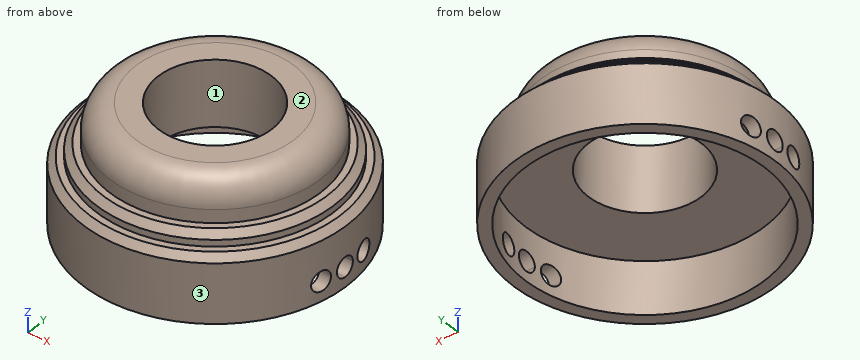
from build123d import *

# Parameters (mm, degrees)
F0_R          = 10
F0_R_2        = 9.1
F1_DEPTH      = 4
F2_R          = 0.75
F3_DEPTH      = 25
F3_DEPTH_BACK = 25
F4_R          = 10
F4_R_2        = 9.1
F4_R_3        = 9
F4_R_4        = 8
F4_R_5        = 4.3
F5_DEPTH      = 1
F6_DEPTH      = 2
F7_DEPTH      = 5
F8_SIZE       = 0.5
F9_R          = 2


with BuildPart() as f1:
    # F0 (on Top) → F1 (new body)
    with BuildSketch(Plane.XY):
        Circle(F0_R)
        Circle(F0_R_2, mode=Mode.SUBTRACT)
    extrude(amount=F1_DEPTH)

    # F2 (on Right) → F3 (cut, two sides)
    with BuildSketch(Plane.YZ) as f3_sk:
        with BuildLine():
            ThreePointArc((-0.75, 1.5), (-0.5303300859, 0.9696699141), (0, 0.75))
            Line((0, 0.75), (0, 1.5))
            Line((0, 1.5), (-0.75, 1.5))
        make_face()
        with BuildLine():
            Line((0, 1.5), (0, 0.75))
            ThreePointArc((0, 0.75), (0.5303300859, 0.9696699141), (0.75, 1.5))
            Line((0.75, 1.5), (0, 1.5))
        make_face()
        with BuildLine():
            Line((-0.75, 1.5), (0, 1.5))
            Line((0, 1.5), (0.75, 1.5))
            ThreePointArc((0.75, 1.5), (0, 2.25), (-0.75, 1.5))
        make_face()
        with Locations((-2, 1.5)):
            Circle(F2_R)
        with BuildLine():
            ThreePointArc((2.75, 1.5), (2, 2.25), (1.25, 1.5))
            ThreePointArc((1.25, 1.5), (2, 0.75), (2.75, 1.5))
        make_face()
    extrude(amount=-F3_DEPTH, mode=Mode.SUBTRACT)
    extrude(f3_sk.sketch, amount=F3_DEPTH_BACK, mode=Mode.SUBTRACT)

    # F4 (on face) → F5 (join)
    with BuildSketch(Plane.XY.offset(4)):
        Circle(F4_R)
        Circle(F4_R_2, mode=Mode.SUBTRACT)
        Circle(F4_R_2)
        Circle(F4_R_3, mode=Mode.SUBTRACT)
        Circle(F4_R_3)
        Circle(F4_R_4, mode=Mode.SUBTRACT)
        Circle(F4_R_4)
        Circle(F4_R_5, mode=Mode.SUBTRACT)
    extrude(amount=F5_DEPTH)

    # F4 (on face) → F6 (join)
    with BuildSketch(Plane.XY.offset(4)):
        Circle(F4_R_3)
        Circle(F4_R_4, mode=Mode.SUBTRACT)
        Circle(F4_R_4)
        Circle(F4_R_5, mode=Mode.SUBTRACT)
    extrude(amount=F6_DEPTH)

    # F4 (on face) → F7 (join)
    with BuildSketch(Plane.XY.offset(4)):
        Circle(F4_R_4)
        Circle(F4_R_5, mode=Mode.SUBTRACT)
    extrude(amount=F7_DEPTH)

    # F8
    f8_edges = [f1.edges().sort_by_distance(p)[0] for p in [
        (-10, 0, 5),
        (-9, 0, 6),
    ]]
    chamfer(f8_edges, length=F8_SIZE)

    # F9
    f9_edges = [f1.edges().sort_by_distance(p)[0] for p in [
        (-8, 0, 9),
    ]]
    fillet(f9_edges, radius=F9_R)


solid = f1.part
Build history of the part. All positions in model axes, mm. Face numbers are marked on the shaded views. Coordinates: 2 decimals unless noted, no trailing zeros. Write each loop counter-clockwise with the first axis right and the second up, starting at its lowest first coordinate (ties: lowest second). Pieces come first, ordered by that corner, then holes. Notation, with made-up numbers: (81, -24.75) -> (139, -24.75) arc R17 ccw to (139, -11.75) -> close; hole circle Ø11 at (19.5, 22.25). An arc over 180 degrees is marked (long way). Use CSV: the item, a comma, the result in double quotes. Start each with the question number.
Q1. Pull direction X, two halves, no side cores. Call the marked faces 1, 2 and 3: released by +X, released by -X, zero draft, split by the parting line, or undercut.
Q2. Drill centre lines: probe 1 along Z at (x, y) = (9.15, 2); probe 2 along Y at (x, z) = (0, 6.4); probe 3 along Y at (x, z) = (9.15, 1.5). Where is each one in solid material? Low to high.
Q3. Cut at B-B, the plane z = 0.5. List the corners of the cut face in (x, y), then the cut area to 3 significant figures.
Q4. Cut at D-D, the plane z = 7.75. List the corners of the cut face in (x, y), then the cut area to 3 significant figures.
Q5. Cut at A-A, the plane x = 0. List the corners of the cut face in (y, z).
Q6. Flat gauge pins, fed straight in: pin 1 Ø1.5 at (y, z) = (0, 6) entering from +X; pin 2 Ø1 at (y, z) = (2.5, 5) entering from +X; pin 3 Ø1.5 at (x, z) = (7.5, 5.5) entering from +Y. Where does each tip first touch, or does it go through?
Q7. Cut at C-C, the plane y = -2. State how many separate pieces and enclosed holes the cut face has, then the cut area to 3 significant figures.
Checked values:
1,face 1,"undercut"
1,face 2,"zero draft"
1,face 3,"split by the parting line"
2,probe 1,"z = 0 to 0.75, 2.25 to 5"
2,probe 2,"y = -8 to -4.3, 4.3 to 8"
2,probe 3,"y = -4.03 to -2.75, -1.25 to -0.75, 0.75 to 1.25, 2.75 to 4.03"
3,outline,"circle Ø20 at (0, 0); hole circle Ø18.2 at (0, 0)"
3,area,"54.0 mm²"
4,outline,"circle Ø15.71 at (0, 0); hole circle Ø8.6 at (0, 0)"
4,area,"136 mm²"
5,outline,"(-10, 0) -> (-9.1, 0) -> (-9.1, 4) -> (-4.3, 4) -> (-4.3, 9) -> (-6, 9) arc R2 ccw to (-8, 7) -> (-8, 6) -> (-8.5, 6) -> (-9, 5.5) -> (-9, 5) -> (-9.5, 5) -> (-10, 4.5) -> close; (4.3, 4) -> (9.1, 4) -> (9.1, 0) -> (10, 0) -> (10, 4.5) -> (9.5, 5) -> (9, 5) -> (9, 5.5) -> (8.5, 6) -> (8, 6) -> (8, 7) arc R2 ccw to (6, 9) -> (4.3, 9) -> close"
6,pin 1,"stops at x = 9"
6,pin 2,"stops at x = 9.7"
6,pin 3,"stops at y = 6.52"
7,separate pieces,"4"
7,enclosed holes,"0"
7,area,"47.9 mm²"
